from build123d import *

# Parameters (mm, degrees)
F0_W     = 1.27
F0_H     = 25.4
F1_DEPTH = 1
F2_W     = 25.4
F2_H     = 14.24
F2_R     = 0.635
F2_H_2   = 1
F3_DEPTH = 3.81
F5_R     = 12.69999
F6_R     = 12.69999
F7_R     = 1.26999
F7_2_R   = 1.26999
F8_DEPTH = 0.0889


# Not quite as in the source:
# - a fillet or chamfer is up to 0.001 mm smaller than in the source, because OpenCascade refuses the exact size


with BuildPart() as f1:
    # F0 (on Top) → F1 (new body)
    with BuildSketch(Plane.XY):
        with Locations((-12.065, 0)):
            Rectangle(F0_W, F0_H)
    extrude(amount=F1_DEPTH)

    # F7 (radius 1.27 in the source; OpenCascade refuses exactly that, so slightly less here)
    f7_edges = [f1.edges().sort_by_distance(p)[0] for p in [
        (-12.7, -12.7, 0.5),
        (-12.7, 12.7, 0.5),
    ]]
    fillet(f7_edges, radius=F7_R)

    # F8 (add): a face of the model
    f8_faces = [f1.faces().sort_by_distance(p)[0] for p in [
        (-11.43, 0, 0.5),
    ]]


with BuildPart() as f1b:
    # F0 (on Top) → F1, piece 2 (new body)
    with BuildSketch(Plane.XY):
        with Locations((12.065, 0)):
            Rectangle(F0_W, F0_H)
    extrude(amount=F1_DEPTH)

    # F7#2 (radius 1.27 in the source; OpenCascade refuses exactly that, so slightly less here)
    f7_2_edges = [f1b.edges().sort_by_distance(p)[0] for p in [
        (12.7, -12.7, 0.5),
        (12.7, 12.7, 0.5),
    ]]
    fillet(f7_2_edges, radius=F7_2_R)


with BuildPart() as f1c:
    # F0 (on Top) → F1, piece 3 (new body)
    with BuildSketch(Plane.XY):
        with BuildLine():
            Line((0, -12.7), (7.62, -12.7))
            Line((7.62, -12.7), (7.62, 12.7))
            Line((7.62, 12.7), (0, 12.7))
            Line((0, 12.7), (0, 2))
            ThreePointArc((0, 2), (1.4142135624, 1.4142135624), (2, 0))
            ThreePointArc((2, 0), (1.4142135624, -1.4142135624), (0, -2))
            Line((0, -2), (0, -12.7))
        make_face()
        with BuildLine():
            Line((-7.62, -12.7), (0, -12.7))
            Line((0, -12.7), (0, -2))
            ThreePointArc((0, -2), (-2, 0), (0, 2))
            Line((0, 2), (0, 12.7))
            Line((0, 12.7), (-7.62, 12.7))
            Line((-7.62, 12.7), (-7.62, -12.7))
        make_face()
    extrude(amount=F1_DEPTH)


with BuildPart() as f3:
    # F2 (on face) → F3 (new body)
    with BuildSketch(Plane(origin=(11.43, 0, 0), x_dir=(0, -1, 0), z_dir=(-1, 0, 0))):
        with Locations((0, -7.12)):
            Rectangle(F2_W, F2_H)
        with Locations((0, -12.7)):
            Circle(F2_R, mode=Mode.SUBTRACT)
        with Locations((0, 0.5)):
            Rectangle(F2_W, F2_H_2)
    extrude(amount=F3_DEPTH)


with BuildPart() as f4_1:
    # F4: copy of F3
    add(f3.part.moved(Location((-18.961354, 0, 0))))

    # F6 (radius 12.7 in the source; OpenCascade refuses exactly that, so slightly less here)
    f6_edges = [f4_1.edges().sort_by_distance(p)[0] for p in [
        (-9.436354, -12.7, -14.24),
        (-9.436354, 12.7, -14.24),
    ]]
    fillet(f6_edges, radius=F6_R)


with BuildPart() as f3_1:
    add(f3.part)

    # F5 (radius 12.7 in the source; OpenCascade refuses exactly that, so slightly less here)
    f5_edges = [f3_1.edges().sort_by_distance(p)[0] for p in [
        (9.525, -12.7, -14.24),
        (9.525, 12.7, -14.24),
    ]]
    fillet(f5_edges, radius=F5_R)


with BuildPart() as f1_1:
    add(f1.part)

    add(f1b.part)  # F8 merges F1b

    add(f1c.part)  # F8 merges F1c

    add(f3_1.part)  # F8 merges F3

    add(f4_1.part)  # F8 merges F4_1
    extrude(f8_faces, amount=F8_DEPTH)


solid = f1_1.part
Could you check a few things on this model? Use its own coordinates, in mm. A direction names the side the tool comes from. Give positions to 0.01 mm unless a question says otherwise; leave off trailing zeros. Order: outer loops, then holes, each group sorted by start corner. A loop starts at its lowest first (then second) coordinate and runs counter-clockwise, first axis right, second up. Notation, with made-up numbers: (-24.75, 76.5) -> (34.25, 76.5) arc R14 ccw to (34.25, 93.5) -> close; hole circle Ø7 at (-13.75, -15.5). An arc over 180 degrees is marked (long way). Answer in a Markdown table with one row per item. Add a question column.
Item 1: Imagine slicing it at D-D (y = -2.5). List the corners of the cut face in (x, z) for me, and give its area (3 significant figures).
Item 2: For faces 4 (the flat face through (-0.2, -12.7, 0.3)), 5 (the flat face through (0, 3, 0)), 6 (the flat face through (12, 0, 0)), 7 (the flat face through (-12, 0, 0)), 8 (the flat face through (-12.7, -0.2, 0.5)), which set-ups out of +Z, -Z, +X, -X, +Y, -Y let a thin tool reach every point of the face, with its end or its side?
Item 3: Please list where these lines run through material, in increasing order: probe 1 along Z at (x, y) = (8.7, 0) (3 decimals); probe 2 along X at (y, z) = (-5, -12.5); probe 3 along Z at (x, y) = (-6, -10.75).
Item 4: We'd pull the mould along Z, two halves only. Please class faces 1 (the cylindrical face through (-9.41, 0.08, -12.07)), 2 (the flat face through (11.43, 0, -5)), 3 (the cylindrical face through (9.5, -8.9, -10.6)): pulls with the +Z half, pulls with the -Z half, needs draft (parallel to the pull), parting line crosses it, or undercut.
Item 5: Imagine slicing it at C-C (z = -12.7). List the corners of the cut face in (x, y) for me (3 decimals), and give its area (3 significant figures).
Item 6: Imagine slicing it at B-B (z = -10). List the corners of the cut face in (x, y) for me, and give its area (3 significant figures).
Item 7: I'm going to push flat-ended pins straight in: P1, Ø10, axis at x = -3, y = 2.5, coming from the -Z side; P2, Ø6, axis at y = 10, z = -9.5, coming from the +X side; P3, Ø7.5, axis at x = 2.5, y = 2, coming from the -Z side; P4, Ø1.1, axis at y = 0, z = -12.7, coming from the +X side. Where does each tip first touch, or does it pass through?
Result:
| question | item | result |
|---|---|---|
| 1 | outline | (-12.7, 0) -> (-11.34, 0) -> (-11.34, -13.99) -> (-7.53, -13.99) -> (-7.53, 0) -> (7.62, 0) -> (7.62, -13.99) -> (11.43, -13.99) -> (11.43, 0) -> (12.7, 0) -> (12.7, 1) -> (-12.7, 1) -> close |
| 1 | area | 132 mm2 |
| 2 | face 4 | +Z, -Z, +X, -X, -Y |
| 2 | face 5 | -Z, +Y, -Y |
| 2 | face 6 | -Z, +X, +Y, -Y |
| 2 | face 7 | -Z, -X, +Y, -Y |
| 2 | face 8 | +Z, -Z, -X, +Y, -Y |
| 3 | probe 1 | -14.24 to -13.335, -12.065 to 1 |
| 3 | probe 2 | -11.34 to -7.53, 7.62 to 11.43 |
| 3 | probe 3 | 0 to 1 |
| 4 | face 1 | undercut |
| 4 | face 2 | needs draft |
| 4 | face 3 | pulls with the -Z half |
| 5 | outline | (-11.341, -6.062) -> (-7.531, -6.062) -> (-7.531, -0.635) -> (-11.341, -0.635) -> close; (-11.341, 0.635) -> (-7.531, 0.635) -> (-7.531, 6.062) -> (-11.341, 6.062) -> close; (7.62, -6.062) -> (11.43, -6.062) -> (11.43, -0.635) -> (7.62, -0.635) -> close; (7.62, 0.635) -> (11.43, 0.635) -> (11.43, 6.062) -> (7.62, 6.062) -> close |
| 5 | area | 82.7 mm2 |
| 6 | outline | (-11.34, -9.47) -> (-7.53, -9.47) -> (-7.53, 9.47) -> (-11.34, 9.47) -> close; (7.62, -9.47) -> (11.43, -9.47) -> (11.43, 9.47) -> (7.62, 9.47) -> close |
| 6 | area | 144 mm2 |
| 7 | P1 | z = -14.23 |
| 7 | P2 | x = 11.43 |
| 7 | P3 | z = 0 |
| 7 | P4 | through |
